Check sheet for the modelled part. Datum: model origin and axes. Units: mm. Face numbers are marked on the shaded views. A direction names the side the tool comes from. Round coordinates to 2 decimals unless told otherwise and drop trailing zeros. Loops run counter-clockwise (first coordinate to the right, second up) from the corner with the lowest first, then second, coordinate; pieces in that order, holes last. Notation, with made-up numbers: (1, 20) -> (24, 20) arc R33 cw to (24, 51) -> close; hole circle Ø9 at (-25.5, -26). An arc over 180 degrees is marked (long way). Return JSON: item names as keys, results as strings.
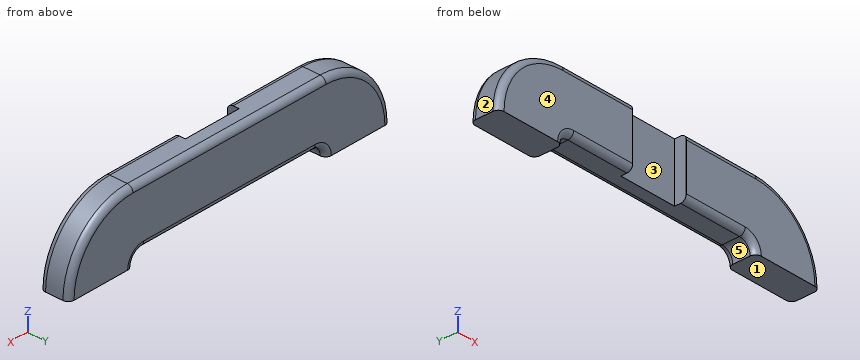
from build123d import *

# Parameters (mm, degrees)
F0_W         = 90
F0_H         = 50
F1_DEPTH     = 25
F2_R         = 59.99999
F3_R         = 9.99999
F4_R         = 9.99999
F5_R         = 59.99999
F6_T1_DEPTH  = 12.50001
F6_T3_DEPTH  = 180.00002
F6_T6_ANGLE  = 90
F6_T8_ANGLE  = 90
F7_T1_DEPTH  = 12.50001
F7_T3_DEPTH  = 180.00002
F7_T6_ANGLE  = 90
F7_T8_ANGLE  = 90
F8_T1_DEPTH  = 160.00002
F8_T3_DEPTH  = 12.50001
F8_T6_ANGLE  = 90
F8_T8_ANGLE  = 90
F8_T10_ANGLE = 90
F8_T12_ANGLE = 90
F9_W         = 50
F9_H         = 5
F9_H_2       = 40
F10_DEPTH    = 10
F13_W        = 50
F13_H        = 10
F14_DEPTH    = 60.001
F16_DEPTH    = 10


# Not quite as in the source:
# - a fillet or chamfer that OpenCascade refuses, or shapes differently, is made with other operations: its cross-section is extruded or revolved along the edge and cut away or added
# - a fillet or chamfer is up to 0.001 mm smaller than in the source, because OpenCascade refuses the exact size


with BuildPart() as f1:
    # F0 (on Front) → F1 (new body)
    with BuildSketch(Plane.XZ):
        with Locations((45, 0)):
            Rectangle(F0_W, F0_H)
        Polygon((150, 25), (90, 25), (90, -25), (90, -35), (150, -35), align=None)
        with Locations((-45, 0)):
            Rectangle(F0_W, F0_H)
        Polygon((-90, -25), (-90, 25), (-150, 25), (-150, -35), (-90, -35), align=None)
    extrude(amount=F1_DEPTH)

    # F2 (radius 60 in the source; OpenCascade refuses exactly that, so slightly less here)
    f2_edges = [f1.edges().sort_by_distance(p)[0] for p in [
        (-150, -12.5, 25),
    ]]
    fillet(f2_edges, radius=F2_R)

    # F3 (radius 10 in the source; OpenCascade refuses exactly that, so slightly less here)
    f3_edges = [f1.edges().sort_by_distance(p)[0] for p in [
        (-90, -12.5, -25),
    ]]
    fillet(f3_edges, radius=F3_R)

    # F4 (radius 10 in the source; OpenCascade refuses exactly that, so slightly less here)
    f4_edges = [f1.edges().sort_by_distance(p)[0] for p in [
        (90, -12.5, -25),
    ]]
    fillet(f4_edges, radius=F4_R)

    # F5 (radius 60 in the source; OpenCascade refuses exactly that, so slightly less here)
    f5_edges = [f1.edges().sort_by_distance(p)[0] for p in [
        (150, -12.5, 25),
    ]]
    fillet(f5_edges, radius=F5_R)

    # F6: fillet of radius 5 on 1 edges, made by hand

    # F6_s2 → F6_t1 (cut)
    with BuildSketch(Plane.XY.offset(-47.5)):
        with BuildLine():
            ThreePointArc((150, -20), (148.5355339059, -23.5355339059), (145, -25))
            Line((145, -25), (150, -25))
            Line((150, -25), (150, -20))
        make_face()
        with BuildLine():
            ThreePointArc((-150, -20), (-148.5355339059, -23.5355339059), (-145, -25))
            Line((-145, -25), (-150, -25))
            Line((-150, -25), (-150, -20))
        make_face()
    extrude(amount=F6_T1_DEPTH, mode=Mode.SUBTRACT)

    # F6_s4 → F6_t3 (cut)
    with BuildSketch(Plane.YZ.offset(-90.00001)):
        with BuildLine():
            ThreePointArc((-20, 25), (-23.5355339059, 23.5355339059), (-25, 20))
            Line((-25, 20), (-25, 25))
            Line((-25, 25), (-20, 25))
        make_face()
    extrude(amount=F6_T3_DEPTH, mode=Mode.SUBTRACT)

    # F6_s5 → F6_t6 (revolve, cut)
    with BuildSketch(Plane.XY.offset(-34.99999)):
        with BuildLine():
            ThreePointArc((150, -20), (148.5355339059, -23.5355339059), (145, -25))
            Line((145, -25), (150, -25))
            Line((150, -25), (150, -20))
        make_face()
    revolve(axis=Axis((90.00001, -25, -34.99999), (0, -1, 0)), revolution_arc=F6_T6_ANGLE, mode=Mode.SUBTRACT)

    # F6_s7 → F6_t8 (revolve, cut)
    with BuildSketch(Plane.YZ.offset(-90.00001)):
        with BuildLine():
            ThreePointArc((-20, 25), (-23.5355339059, 23.5355339059), (-25, 20))
            Line((-25, 20), (-25, 25))
            Line((-25, 25), (-20, 25))
        make_face()
    revolve(axis=Axis((-90.00001, -25, -34.99999), (0, -1, 0)), revolution_arc=F6_T8_ANGLE, mode=Mode.SUBTRACT)

    # F7: fillet of radius 5 on 1 edges, made by hand

    # F7_s2 → F7_t1 (cut)
    with BuildSketch(Plane.XY.offset(-47.5)):
        with BuildLine():
            ThreePointArc((145, 0), (148.5355339059, -1.4644660941), (150, -5))
            Line((150, -5), (150, 0))
            Line((150, 0), (145, 0))
        make_face()
        with BuildLine():
            ThreePointArc((-145, 0), (-148.5355339059, -1.4644660941), (-150, -5))
            Line((-150, -5), (-150, 0))
            Line((-150, 0), (-145, 0))
        make_face()
    extrude(amount=F7_T1_DEPTH, mode=Mode.SUBTRACT)

    # F7_s4 → F7_t3 (cut)
    with BuildSketch(Plane.YZ.offset(-90.00001)):
        with BuildLine():
            ThreePointArc((0, 20), (-1.4644660941, 23.5355339059), (-5, 25))
            Line((-5, 25), (0, 25))
            Line((0, 25), (0, 20))
        make_face()
    extrude(amount=F7_T3_DEPTH, mode=Mode.SUBTRACT)

    # F7_s5 → F7_t6 (revolve, cut)
    with BuildSketch(Plane.XY.offset(-34.99999)):
        with BuildLine():
            ThreePointArc((145, 0), (148.5355339059, -1.4644660941), (150, -5))
            Line((150, -5), (150, 0))
            Line((150, 0), (145, 0))
        make_face()
    revolve(axis=Axis((90.00001, 0, -34.99999), (0, -1, 0)), revolution_arc=F7_T6_ANGLE, mode=Mode.SUBTRACT)

    # F7_s7 → F7_t8 (revolve, cut)
    with BuildSketch(Plane.YZ.offset(-90.00001)):
        with BuildLine():
            ThreePointArc((0, 20), (-1.4644660941, 23.5355339059), (-5, 25))
            Line((-5, 25), (0, 25))
            Line((0, 25), (0, 20))
        make_face()
    revolve(axis=Axis((-90.00001, 0, -34.99999), (0, -1, 0)), revolution_arc=F7_T8_ANGLE, mode=Mode.SUBTRACT)

    # F8: fillet of radius 5 on 2 edges, made by hand

    # F8_s2 → F8_t1 (cut)
    with BuildSketch(Plane.YZ.offset(-80.00001)):
        with BuildLine():
            ThreePointArc((-20, -25), (-23.5355339059, -23.5355339059), (-25, -20))
            Line((-25, -20), (-25, -25))
            Line((-25, -25), (-20, -25))
        make_face()
        with BuildLine():
            ThreePointArc((0, -20), (-1.4644660941, -23.5355339059), (-5, -25))
            Line((-5, -25), (0, -25))
            Line((0, -25), (0, -20))
        make_face()
    extrude(amount=F8_T1_DEPTH, mode=Mode.SUBTRACT)

    # F8_s4 → F8_t3 (cut)
    with BuildSketch(Plane.XY.offset(-47.5)):
        with BuildLine():
            ThreePointArc((90, -20), (91.4644660941, -23.5355339059), (95, -25))
            Line((95, -25), (90, -25))
            Line((90, -25), (90, -20))
        make_face()
        with BuildLine():
            ThreePointArc((-90, -20), (-91.4644660941, -23.5355339059), (-95, -25))
            Line((-95, -25), (-90, -25))
            Line((-90, -25), (-90, -20))
        make_face()
        with BuildLine():
            ThreePointArc((95, 0), (91.4644660941, -1.4644660941), (90, -5))
            Line((90, -5), (90, 0))
            Line((90, 0), (95, 0))
        make_face()
        with BuildLine():
            ThreePointArc((-95, 0), (-91.4644660941, -1.4644660941), (-90, -5))
            Line((-90, -5), (-90, 0))
            Line((-90, 0), (-95, 0))
        make_face()
    extrude(amount=F8_T3_DEPTH, mode=Mode.SUBTRACT)

    # F8_s5 → F8_t6 (revolve, cut)
    with BuildSketch(Plane.YZ.offset(80.00001)):
        with BuildLine():
            ThreePointArc((0, -20), (-1.4644660941, -23.5355339059), (-5, -25))
            Line((-5, -25), (0, -25))
            Line((0, -25), (0, -20))
        make_face()
    revolve(axis=Axis((80.00001, 0, -34.99999), (0, 1, 0)), revolution_arc=F8_T6_ANGLE, mode=Mode.SUBTRACT)

    # F8_s7 → F8_t8 (revolve, cut)
    with BuildSketch(Plane.XY.offset(-34.99999)):
        with BuildLine():
            ThreePointArc((-90, -20), (-91.4644660941, -23.5355339059), (-95, -25))
            Line((-95, -25), (-90, -25))
            Line((-90, -25), (-90, -20))
        make_face()
    revolve(axis=Axis((-80.00001, -25, -34.99999), (0, 1, 0)), revolution_arc=F8_T8_ANGLE, mode=Mode.SUBTRACT)

    # F8_s9 → F8_t10 (revolve, cut)
    with BuildSketch(Plane.YZ.offset(80.00001)):
        with BuildLine():
            ThreePointArc((-20, -25), (-23.5355339059, -23.5355339059), (-25, -20))
            Line((-25, -20), (-25, -25))
            Line((-25, -25), (-20, -25))
        make_face()
    revolve(axis=Axis((80.00001, -25, -34.99999), (0, 1, 0)), revolution_arc=F8_T10_ANGLE, mode=Mode.SUBTRACT)

    # F8_s11 → F8_t12 (revolve, cut)
    with BuildSketch(Plane.XY.offset(-34.99999)):
        with BuildLine():
            ThreePointArc((-95, 0), (-91.4644660941, -1.4644660941), (-90, -5))
            Line((-90, -5), (-90, 0))
            Line((-90, 0), (-95, 0))
        make_face()
    revolve(axis=Axis((-80.00001, 0, -34.99999), (0, 1, 0)), revolution_arc=F8_T12_ANGLE, mode=Mode.SUBTRACT)

    # F9 (on face) → F10 (join)
    with BuildSketch(Plane.XZ.offset(25)):
        with Locations((0, -22.5)):
            Rectangle(F9_W, F9_H)
        with Locations((0, 22.5)):
            Rectangle(F9_W, F9_H)
        Rectangle(F9_W, F9_H_2)
    extrude(amount=-F10_DEPTH)

    # F13 (on face) → F14 (cut, through all)
    with BuildSketch(Plane.XY.offset(25)):
        with Locations((0.0907536596, -19.8229007973)):
            Rectangle(F13_W, F13_H)
    extrude(amount=-F14_DEPTH, mode=Mode.SUBTRACT)

    # F15 (on face) → F16 (cut)
    with BuildSketch(Plane.XZ.offset(25)):
        Polygon((25, 25), (-25, 25), (-25, 20), (-25, -20), (-25, -25), (25, -25), (25, -20), (25, 20), align=None)
    extrude(amount=-F16_DEPTH, mode=Mode.SUBTRACT)


solid = f1.part
Q1. Go/stop test with flat-tipped pins: pin 1 (10 mm diameter, centred on x = 58, y = -16, fed in from -Z); pin 2 (10 mm diameter, centred on y = -19, z = 10, fed in from -X); pin 3 (25 mm diameter, centred on x = 12, z = 7, fed in from -Y); pin 4 (5 mm diameter, centred on x = -29, y = -22, fed in from +Z). Record where each tip stops, or that it passes through.
Results list:
{"pin 1": "z = -25", "pin 2": "x = -134.72", "pin 3": "y = -14.82", "pin 4": "z = 25"}
Q2. Material ranges on line 1 (Z direction, x = -78.5, y = -5.75); line 2 (Y direction, x = -6.5, z = -3.5); line 3 (X direction, y = -21.5, z = -20.5), recorded low to high.
Results list:
{"line 1": "-25 to 25", "line 2": "-14.82 to 0", "line 3": "-147.98 to -25, 25.09 to 147.98"}
Q3. Tool access check on the marked faces 4 and 5. Record the directions out of +Z, -Z, +X, -X, +Y, -Y that give a thin tool (end or side, any length) a straight path to the whole face; none if there is none.
Results list:
{"face 4": "+Z, -Z, +X, -X, -Y", "face 5": "-Z, +Y, -Y"}
Q4. Draft check along X on the marked faces 1, 2 and 3. Enter one of: released by +X, released by -X, zero draft, split by the parting line, or undercut.
Results list:
{"face 1": "zero draft", "face 2": "released by -X", "face 3": "undercut"}
Q5. Section check A-A (x = -33.5). Record the boundary of the cut face in (y, z), then the cut area to 3 significant figures.
Results list:
{"outline": "(-25, -20) arc R5 ccw to (-20, -25) -> (-5, -25) arc R5 ccw to (0, -20) -> (0, 20) arc R5 ccw to (-5, 25) -> (-20, 25) arc R5 ccw to (-25, 20) -> close", "area": "1,230 mm^2"}
